For this review, use the dimensioned drawing (mm, ordinates from the lowest corner) and the shaded views. A direction names the side the tool comes from. Round coordinates to 2 decimals unless told otherwise and drop trailing zeros. Order: outer loops, then holes, each group sorted by start corner. A loop starts at its lowest first (then second) coordinate and runs counter-clockwise, first axis right, second up. Notation, with made-up numbers: (65, 53.5) - (107, 53.5) arc R10 ccw to (107, 66.5) - close; hole circle Ø1 at (-22.5, -8.5). An arc over 180 degrees is marked (long way). Write item = value, one per line.
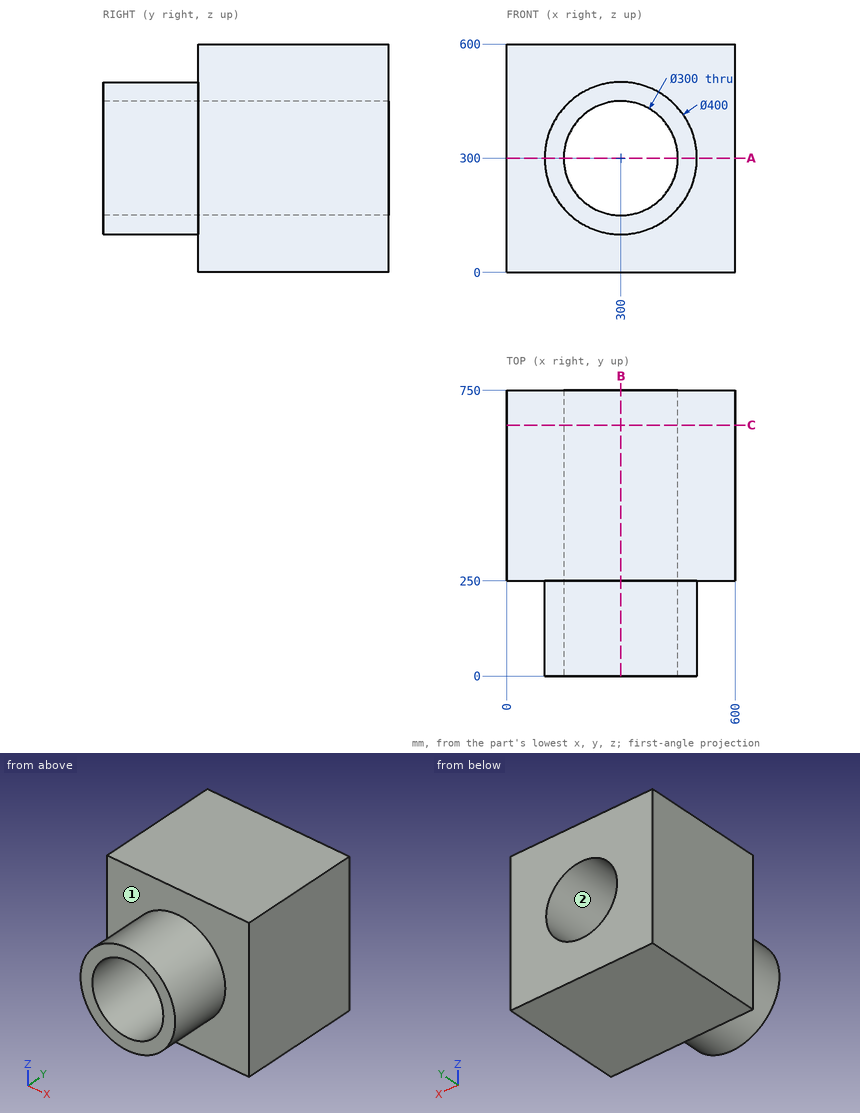
1) We need section A-A on z = 300. Write out the cut boundary in (x, y), and give its area (3 significant figures).
Findings:
outline = (0, 250) - (100, 250) - (100, 0) - (150, 0) - (150, 750) - (0, 750) - close; (450, 0) - (500, 0) - (500, 250) - (600, 250) - (600, 750) - (450, 750) - close
area = 175,000 mm^2
2) Clearance check with flat-ended pins moving along their axes: pin 1 Ø8 at (x, z) = (150, 455.5) entering from -Y; pin 2 Ø8 at (y, z) = (191.5, 251.5) entering from +X; pin 3 Ø3 at (x, y) = (203.5, 466.5) entering from -Z. State where each tip first meets the part, or that it passes through.
Findings:
pin_1 = 250
pin_2 = 494.99
pin_3 = 0
3) For the marked faces 1 and 2, list the 3-axis set-ups (+Z, -Z, +X, -X, +Y, -Y) from which the entire face can be reached by the end or side of a thin tool; tool diameter is ignored.
Findings:
face_1 = -Y
face_2 = +Y, -Y
4) We need section C-C on y = 659. Write out the cut boundary in (x, z).
Findings:
outline = (0, 0) - (600, 0) - (600, 600) - (0, 600) - close; hole circle Ø300 at (300, 300)
5) To check wall thickness, follow L1, parallel to Z at x = 300, y = 579; L2, parallel to Z at x = 300, y = 232; L3, parallel to Y at x = 499, z = 440. State the ranges of each line that lie inside material, in increasing order. Write a range as from..to.
Findings:
L1 = 0..150, 450..600
L2 = 100..150, 450..500
L3 = 250..750
6) We need section B-B on x = 300. Write out the cut boundary in (y, z).
Findings:
outline = (0, 100) - (250, 100) - (250, 0) - (750, 0) - (750, 150) - (0, 150) - close; (0, 450) - (750, 450) - (750, 600) - (250, 600) - (250, 500) - (0, 500) - close
